Design review of the part built by this model. Coordinates are the model's own, in mm. Coordinates: 2 decimals unless noted, no trailing zeros. Write each loop counter-clockwise with the first axis right and the second up, starting at its lowest first coordinate (ties: lowest second). Pieces come first, ordered by that corner, then holes. Notation, with made-up numbers: M 17,21.25 L 23,21.25 A24 cw 23,59.25 Z; hole C 72.25,26.25 d8. An arc over 180 degrees is marked long. Write each question's results on one line, items separated by ' | '. Start each with the question number.
```python
from build123d import *

# Parameters (mm, degrees)
F0_R     = 50.8
F0_R_2   = 4.826
F1_DEPTH = 3.175
F3_DEPTH = 25.4


with BuildPart() as f1:
    # F0 (on Front) → F1 (new body)
    with BuildSketch(Plane.XZ):
        Circle(F0_R)
        with BuildLine():
            Line((-3.175, -31.6174778593), (-3.175, -44.45))
            ThreePointArc((-3.175, -44.45), (-31.5109752705, -31.5109752705), (-44.45, -3.175))
            Line((-44.45, -3.175), (-31.6174778593, -3.175))
            ThreePointArc((-31.6174778593, -3.175), (-22.4693739475, -22.4693739475), (-3.175, -31.6174778593))
        make_face(mode=Mode.SUBTRACT)
        with BuildLine():
            ThreePointArc((-8.001, -3.175), (-6.0867325389, -6.0867325389), (-3.175, -8.001))
            Line((-3.175, -8.001), (-3.175, -18.9174778593))
            ThreePointArc((-3.175, -18.9174778593), (-13.5637677944, -13.5637677944), (-18.9174778593, -3.175))
            Line((-18.9174778593, -3.175), (-8.001, -3.175))
        make_face(mode=Mode.SUBTRACT)
        Circle(F0_R_2, mode=Mode.SUBTRACT)
        with BuildLine():
            Line((31.6174778593, -3.175), (44.45, -3.175))
            ThreePointArc((44.45, -3.175), (31.5109752705, -31.5109752705), (3.175, -44.45))
            Line((3.175, -44.45), (3.175, -31.6174778593))
            ThreePointArc((3.175, -31.6174778593), (22.4693739475, -22.4693739475), (31.6174778593, -3.175))
        make_face(mode=Mode.SUBTRACT)
        with BuildLine():
            ThreePointArc((3.175, -8.001), (6.0867325389, -6.0867325389), (8.001, -3.175))
            Line((8.001, -3.175), (18.9174778593, -3.175))
            ThreePointArc((18.9174778593, -3.175), (13.5637677944, -13.5637677944), (3.175, -18.9174778593))
            Line((3.175, -18.9174778593), (3.175, -8.001))
        make_face(mode=Mode.SUBTRACT)
        with BuildLine():
            Line((-3.175, 18.9174778593), (-3.175, 8.001))
            ThreePointArc((-3.175, 8.001), (-6.0867325389, 6.0867325389), (-8.001, 3.175))
            Line((-8.001, 3.175), (-18.9174778593, 3.175))
            ThreePointArc((-18.9174778593, 3.175), (-13.5637677944, 13.5637677944), (-3.175, 18.9174778593))
        make_face(mode=Mode.SUBTRACT)
        with BuildLine():
            ThreePointArc((-44.45, 3.175), (-31.5109752705, 31.5109752705), (-3.175, 44.45))
            Line((-3.175, 44.45), (-3.175, 37.9674778593))
            Line((-3.175, 37.9674778593), (-3.175, 31.6174778593))
            ThreePointArc((-3.175, 31.6174778593), (-22.4693739475, 22.4693739475), (-31.6174778593, 3.175))
            Line((-31.6174778593, 3.175), (-44.45, 3.175))
        make_face(mode=Mode.SUBTRACT)
        with BuildLine():
            ThreePointArc((8.001, 3.175), (6.0867325389, 6.0867325389), (3.175, 8.001))
            Line((3.175, 8.001), (3.175, 18.9174778593))
            ThreePointArc((3.175, 18.9174778593), (13.5637677944, 13.5637677944), (18.9174778593, 3.175))
            Line((18.9174778593, 3.175), (8.001, 3.175))
        make_face(mode=Mode.SUBTRACT)
        with BuildLine():
            Line((3.175, 37.9674778593), (3.175, 44.45))
            ThreePointArc((3.175, 44.45), (31.5109752705, 31.5109752705), (44.45, 3.175))
            Line((44.45, 3.175), (31.6174778593, 3.175))
            ThreePointArc((31.6174778593, 3.175), (22.4693739475, 22.4693739475), (3.175, 31.6174778593))
            Line((3.175, 31.6174778593), (3.175, 37.9674778593))
        make_face(mode=Mode.SUBTRACT)
    extrude(amount=F1_DEPTH)

    # F2 (on face) → F3 (cut)
    with BuildSketch(Plane.XZ.offset(3.175)):
        Polygon((-39.8937948048, 44.5096977055), (-53.3885769546, 7.7240979299), (-39.592076093, 7.7240979299), (-8.112732321, 39.0091240406), (-8.5013657808, 53.1942620873), align=None)
        Polygon((7.0348572917, 55.979128927), (7.0348572917, 38.4760089219), (40.1488728821, 8.9099211618), (41.2437692285, 8.9099211618), (41.2437692285, 11.4161195233), (53.2457668566, 13.9619985828), (46.2986193597, 36.3472476602), align=None)
        Polygon((41.2437692285, 11.4161195233), (41.2437692285, 8.9099211618), (54.8136532307, 8.9099211618), (53.2457668566, 13.9619985828), align=None)
        Polygon((54.8136532307, 8.9099211618), (41.2437692285, 8.9099211618), (41.2437692285, -6.7063555237), (56.2328249216, -6.7009725608), (55.2191524148, -9.5701087266), (60.481145978, -9.5701087266), (60.481145978, 15.4967764392), (53.2457668566, 13.9619985828), align=None)
        Polygon((41.2437692285, -9.5701087266), (41.2437692285, -6.7063555237), (39.6758913994, -6.7069185898), (9.4001442194, -39.3419340253), (9.4001442194, -54.716296494), (44.45, -40.0515161455), (55.2191524148, -9.5701087266), align=None)
        Polygon((56.2328249216, -6.7009725608), (41.2437692285, -6.7063555237), (41.2437692285, -9.5701087266), (55.2191524148, -9.5701087266), align=None)
        Polygon((-8.001, -54.6349138021), (-8.3070490509, -38.0337389297), (-39.696149528, -8.001), (-54.2215406895, -8.001), (-44.45, -37.7750843763), align=None)
    extrude(amount=-F3_DEPTH, mode=Mode.SUBTRACT)


solid = f1.part
```
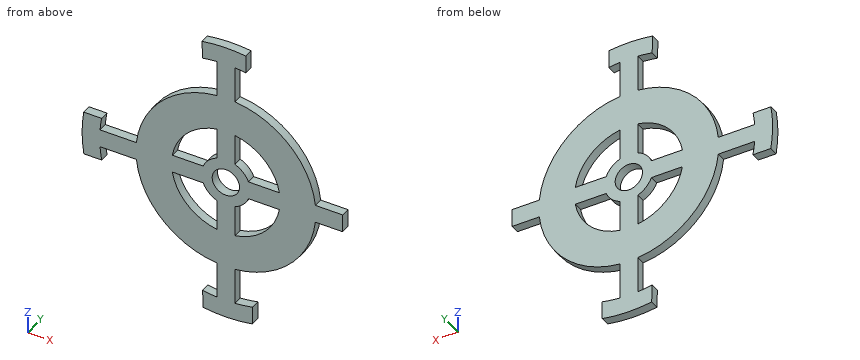
Item 1: We need section B-B on x = 0. State the section outline as (y, z) points (3 decimals).
Item 2: Insertion check: pin 1 Ø1.6 at (y, z) = (-1, -40.5) entering from -X (3 decimals); pin 2 Ø1 at (y, z) = (-2, -48) entering from +X; pin 3 Ø1.6 at (y, z) = (-1, 12.5) entering from +X. Each pin has a flat end and moves straight along its axis. Give the tip position at first contact, or say it passes through.
Item 3: We need section D-D on z = 40.5. State the section outline as (x, y) points (3 decimals), then the cut area to 3 significant figures.
Item 4: Wall thickness on L1, parallel to Z at x = 0, y = -2.5; L2, parallel to X at y = -0.4, z = -3.5; L3, parallel to X at y = -2.1, z = 16.5 (3 decimals): over which ranges is each line inside the solid? List them lowest first.
Item 5: We need section C-C on y = -1.85. Count the separate pieces of the cut face and the enclosed holes in it, then the cut area to 3 significant figures.
Item 6: We need section A-A on z = 0. State the section outline as (x, y) points (3 decimals).
Answer:
1) outline: M -3.175,-50.8 L 0,-50.8 L 0,-4.826 L -3.175,-4.826 Z; M -3.175,4.826 L 0,4.826 L 0,50.8 L -3.175,50.8 Z
2) pin 1: stops at x = -3.175 | pin 2: stops at x = 9.4 | pin 3: stops at x = 29.54
3) outline: M -3.175,-3.175 L 3.175,-3.175 L 3.175,0 L -3.175,0 Z | area: 20.2 mm^2
4) L1: z = -50.8 to -4.83, 4.83 to 50.8 | L2: x = -50.68 to -44.43, -31.58 to -18.86, -7.86 to -3.32, 3.32 to 7.86, 18.86 to 31.58 | L3: x = -27.157 to -9.783, -3.175 to 3.175, 9.783 to 27.157
5) separate pieces: 1 | enclosed holes: 5 | area: 3,060 mm^2
6) outline: M -50.8,-3.175 L -4.826,-3.175 L -4.826,0 L -50.8,0 Z; M 4.826,-3.175 L 41.244,-3.175 L 41.244,0 L 4.826,0 Z
